```python
from build123d import *

# Parameters (mm, degrees)
Y_KSEKLIK_EKSTR_ZYON1_DEPTH = 10
IZIM2_R                     = 1.7
KES_EKSTR_ZYON1_DEPTH       = 47
IZIM3_W                     = 10
IZIM3_H                     = 5
Y_KSEKLIK_EKSTR_ZYON2_DEPTH = 30
KES_EKSTR_ZYON2_DEPTH       = 31
KES_EKSTR_ZYON2_DEPTH_BACK  = 31
IZIM4_R                     = 1.75


with BuildPart() as part:
    # Çizim1 → Yükseklik-Ekstrüzyon1 (new body)
    with BuildSketch(Plane.XY):
        Polygon((0, 0), (35, 0), (35, -37.5), (0, -37.5), (0, -32.5), (30, -32.5), (30, -5), (0, -5), align=None)
    extrude(amount=Y_KSEKLIK_EKSTR_ZYON1_DEPTH)

    # Çizim2 → Kes-Ekstrüzyon1 (cut)
    with BuildSketch(Plane(origin=(0, 0, 0), x_dir=(1, 0, 0), z_dir=(0, 1, 0))):
        with Locations(Location((5.8, -5, 0), (0, 0, 270))):
            Circle(IZIM2_R)
    extrude(amount=-KES_EKSTR_ZYON1_DEPTH, mode=Mode.SUBTRACT)

    # Çizim3 → Yükseklik-Ekstrüzyon2 (add)
    with BuildSketch(Plane.ZY.offset(-30)):
        with Locations((5, -18)):
            Rectangle(IZIM3_W, IZIM3_H)
    extrude(amount=Y_KSEKLIK_EKSTR_ZYON2_DEPTH)

    # Çizim4 → Kes-Ekstrüzyon2 (cut, two sides: drawn at the far end of the back side and taken through both)
    with BuildSketch(Plane(origin=(0, -15.5, 0), x_dir=(1, 0, 0), z_dir=(0, 1, 0)).offset(-KES_EKSTR_ZYON2_DEPTH_BACK)):
        with Locations(Location((5.8, -5, 0), (0, 0, 90))):
            Circle(IZIM4_R)
    extrude(amount=KES_EKSTR_ZYON2_DEPTH + KES_EKSTR_ZYON2_DEPTH_BACK, mode=Mode.SUBTRACT)


solid = part.part
```
Source: CAD feature listing. Evaluate the final solid. Frame: model axes, mm. A direction names the side the tool comes from. Coordinates: 2 decimals unless noted, no trailing zeros. Loops run counter-clockwise (first coordinate to the right, second up) from the corner with the lowest first, then second, coordinate; pieces in that order, holes last. Notation, with made-up numbers: M -38,44.25 L -23,44.25 A27 cw -23,60.25 Z; hole C 11,-29.5 d7. An arc over 180 degrees is marked long. Use a Markdown table: item, result. Add a question column.
Q1. First-contact query: pin 1 (6 mm diameter, centred on x = 28.5, z = 7, fed in from +Y). Flat tip, straight axial feed; report the tip coordinate or a pass-through.
Q2. Draft query along X for faces 3 (the flat face through (15, -5, 5)), 4 (the flat face through (30, -10, 5)), 5 (the cylindrical face through (7.51, -18.04, 5.38)), 6 (the cylindrical face through (7.51, -35.03, 5.38)). Return one class per face: pulls with the +X half, pulls with the -X half, needs draft (parallel to the pull), parting line crosses it, or undercut.
Q3. Section query A-A, the plane x = 5.8. Return loops of the section in (y, z), and give its area (3 significant figures).
Q4. Material intervals for L1, parallel to Y at x = 18, z = 8.5; L2, parallel to X at y = -35.8, z = 5; L3, parallel to X at y = -12, z = 6, sorted ascending.
Q5. Section query C-C, the plane y = -35. Return loops of the section in (x, z), and give its area (3 significant figures).
Q6. Access query for faces 1 (the flat face through (0, -35, 5)), 2 (the flat face through (15, -32.5, 5)). Directions: +Z, -Z, +X, -X, +Y, -Y. A direction counts if a zero-diameter tool reaches every point of the face in a straight line with its end or side. Return the directions, or none.
Q7. Section query D-D, the plane x = 24.5. Return loops of the section in (y, z), and give its area (3 significant figures).
Q8. Section query B-B, the plane z = 5. Return loops of the section in (x, y).
Result:
| question | item | result |
|---|---|---|
| 1 | pin 1 | stops at y = 0 |
| 2 | face 3 | needs draft |
| 2 | face 4 | pulls with the -X half |
| 2 | face 5 | undercut |
| 2 | face 6 | undercut |
| 3 | outline | M -37.5,0 L -32.5,0 L -32.5,3.25 L -37.5,3.25 Z; M -37.5,6.75 L -32.5,6.75 L -32.5,10 L -37.5,10 Z; M -20.5,0 L -15.5,0 L -15.5,3.25 L -20.5,3.25 Z; M -20.5,6.75 L -15.5,6.75 L -15.5,10 L -20.5,10 Z; M -5,0 L 0,0 L 0,3.25 L -5,3.25 Z; M -5,6.75 L 0,6.75 L 0,10 L -5,10 Z |
| 3 | area | 97.5 mm2 |
| 4 | L1 | y = -37.5 to -32.5, -20.5 to -15.5, -5 to 0 |
| 4 | L2 | x = 0 to 4.05, 7.55 to 35 |
| 4 | L3 | x = 30 to 35 |
| 5 | outline | M 0,0 L 35,0 L 35,10 L 0,10 Z; hole C 5.8,5 d3.5 |
| 5 | area | 340 mm2 |
| 6 | face 1 | +Z, -Z, -X, +Y, -Y |
| 6 | face 2 | +Z, -Z, -X |
| 7 | outline | M -37.5,0 L -32.5,0 L -32.5,10 L -37.5,10 Z; M -20.5,0 L -15.5,0 L -15.5,10 L -20.5,10 Z; M -5,0 L 0,0 L 0,10 L -5,10 Z |
| 7 | area | 150 mm2 |
| 8 | outline | M 0,-37.5 L 4.05,-37.5 L 4.05,-32.5 L 0,-32.5 Z; M 0,-20.5 L 4.05,-20.5 L 4.05,-15.5 L 0,-15.5 Z; M 0,-5 L 4.05,-5 L 4.05,0 L 0,0 Z; M 7.55,-37.5 L 35,-37.5 L 35,0 L 7.55,0 L 7.55,-5 L 30,-5 L 30,-15.5 L 7.55,-15.5 L 7.55,-20.5 L 30,-20.5 L 30,-32.5 L 7.55,-32.5 Z |
